Can you work these out from the model? Positions are in its coordinate system, mm. Face numbers are marked on the shaded views. A direction names the side the tool comes from. Give positions to 0.01 mm unless a question says otherwise; leave off trailing zeros. Write each loop counter-clockwise with the first axis right and the second up, starting at its lowest first coordinate (ties: lowest second). Pieces come first, ordered by that corner, then holes.
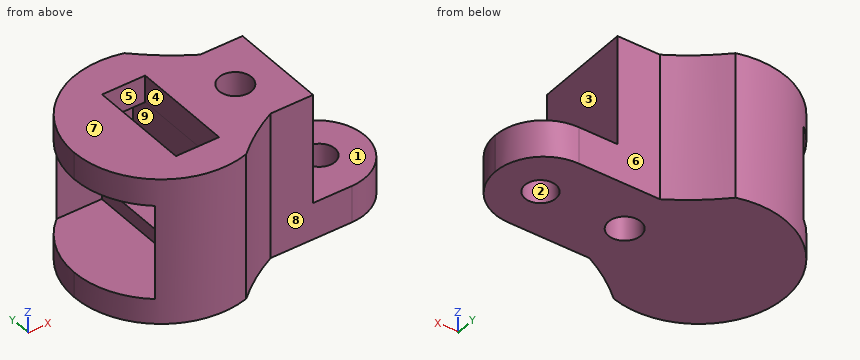
from build123d import *

# Parameters (mm, degrees)
EXTRUDE_1_DEPTH      = 2.2
EXTRUDE_2_DEPTH      = 3.25
SKETCH_3_W           = 50
SKETCH_3_H           = 10.05
EXTRUDE_3_DEPTH      = 3.25
CUT_EXTRUDE_1_DEPTH  = 30
EXTRUDE_4_REACH      = 56.389
SKETCH_6_R           = 5.025
SKETCH_8_R           = 1.675
SKETCH_8_R_2         = 0.84
CUT_EXTRUDE_3_DEPTH  = 55
SKETCH_9_W           = 28.473000816
SKETCH_9_H           = 14.532409192
CUT_EXTRUDE_4_DEPTH  = 3
EXTRUDE_5_DEPTH      = 2.45
SKETCH_11_W          = 12.614203935
SKETCH_11_H          = 10.05
EXTRUDE_6_DEPTH      = 3
SKETCH_12_W          = 36.628466797
SKETCH_12_H          = 15.348537224
CUT_EXTRUDE_5_DEPTH  = 10
SKETCH_13_W          = 5.35
SKETCH_13_H          = 5.35
CUT_EXTRUDE_6_DEPTH  = 14
SKETCH_14_R          = 1.1
CUT_EXTRUDE_7_DEPTH  = 14
SKETCH_15_R          = 1.1
CUT_EXTRUDE_8_DEPTH  = 10
SKETCH_16_R          = 1.625
EXTRUDE_7_DEPTH      = 5.7
SKETCH_17_W          = 19.923143876
SKETCH_17_H          = 15.083058075
CUT_EXTRUDE_9_DEPTH  = 3
SKETCH_18_R          = 1.675
SKETCH_18_R_2        = 1.6
CUT_EXTRUDE_10_DEPTH = 6
CUT_EXTRUDE_11_DEPTH = 10
EXTRUDE_8_DEPTH      = 9.5
EXTRUDE_9_DEPTH      = 15.2
SKETCH_23_W          = 14.793785908
SKETCH_23_H          = 11.59723546
CUT_EXTRUDE_12_DEPTH = 9
SKETCH_25_R          = 1.6
SKETCH_25_R_2        = 1.673969756
CUT_EXTRUDE_13_DEPTH = 20
FILLET_1_R           = 5
SKETCH_26_W          = 0.925753523
SKETCH_26_H          = 16.271734405
EXTRUDE_10_DEPTH     = 15
SKETCH_27_W          = 9.8
SKETCH_27_H          = 13.8
CUT_EXTRUDE_14_DEPTH = 12
SKETCH_28_W          = 4.460954542
SKETCH_28_H          = 10.524407061
CUT_EXTRUDE_15_DEPTH = 12
SKETCH_29_W          = 0.925753523
SKETCH_29_H          = 16.271734405
CUT_EXTRUDE_16_DEPTH = 18
SKETCH_30_W          = 1.5
SKETCH_30_H          = 13.8
EXTRUDE_11_DEPTH     = 3.25


with BuildPart() as part:
    # 草图1 → 凸台-拉伸1 (new body)
    with BuildSketch(Plane.XY):
        with BuildLine():
            Line((1.539836705, 12.851012384), (15.55297303, 14.251012384))
            ThreePointArc((15.55297303, 14.251012384), (17.193415997, 16.063512384), (15.55297303, 17.876012384))
            Line((15.55297303, 17.876012384), (1.500532553, 18.901012384))
            ThreePointArc((1.500532553, 18.901012384), (0.527100583, 19.384612538), (-0.54702697, 19.551012384))
            Line((-0.54702697, 19.551012384), (-0.54702697, 20.901012384))
            Line((-0.54702697, 20.901012384), (19.51277613, 20.901012384))
            Line((19.51277613, 20.901012384), (41.45297303, 20.901012384))
            Line((41.45297303, 20.901012384), (41.45297303, 10.851012384))
            Line((41.45297303, 10.851012384), (-0.54702697, 10.851012384))
            Line((-0.54702697, 10.851012384), (-0.54702697, 12.201012384))
            ThreePointArc((-0.54702697, 12.201012384), (0.54584768, 12.367273294), (1.539836705, 12.851012384))
        make_face()
    extrude(amount=EXTRUDE_1_DEPTH)

    # 草图2 → 凸台-拉伸2 (add)
    with BuildSketch(Plane(origin=(0, 0, 0), x_dir=(-1, 0, 0), z_dir=(0, 0, -1))):
        Polygon((-19.51277613, 10.851012384), (-49.45297303, 10.851012384), (-49.45297303, 20.901012384), (-19.51277613, 20.901012384), (0.54702697, 20.901012384), (0.54702697, 10.851012384), align=None)
    extrude(amount=EXTRUDE_2_DEPTH)

    # 草图3 → 凸台-拉伸3 (add)
    with BuildSketch(Plane.XY.offset(2.2)):
        with Locations((24.45297303, 15.876012384)):
            Rectangle(SKETCH_3_W, SKETCH_3_H)
    extrude(amount=EXTRUDE_3_DEPTH)

    # 草图4 → 切除-拉伸1 (cut, symmetric)
    with BuildSketch(Plane.XY):
        with BuildLine():
            Line((-0.54702697, 19.551012384), (-2.235397712, 16.616091152))
            Line((-2.235397712, 16.616091152), (-1.110896638, 12.310548833))
            Line((-1.110896638, 12.310548833), (-0.54702697, 12.201012384))
            ThreePointArc((-0.54702697, 12.201012384), (0.54584768, 12.367273294), (1.539836705, 12.851012384))
            ThreePointArc((1.539836705, 12.851012384), (2.773180655, 15.88415254), (1.500532553, 18.901012384))
            ThreePointArc((1.500532553, 18.901012384), (0.527100583, 19.384612538), (-0.54702697, 19.551012384))
        make_face()
    extrude(amount=CUT_EXTRUDE_1_DEPTH, both=True, mode=Mode.SUBTRACT)

    # 凸台-拉伸4: up to this face of the body (flat: up to its plane)
    extrude_4_end = Plane(part.part.faces().sort_by_distance((25.407741746, 15.876338503, 5.45))[0])
    # 草图6 → 凸台-拉伸4 (add, up to the picked face)
    with BuildSketch(Plane(origin=(0, 0, -3.25), x_dir=(-1, 0, 0), z_dir=(0, 0, -1)), mode=Mode.PRIVATE) as extrude_4_sk1:
        with Locations(Location((-49.45297303, 15.876012384, 0), (0, 0, 90))):
            Circle(SKETCH_6_R)
    extrude_4_tool1 = split(extrude(extrude_4_sk1.sketch, amount=-EXTRUDE_4_REACH, mode=Mode.PRIVATE), bisect_by=extrude_4_end, keep=Keep.BOTH, mode=Mode.PRIVATE)
    add(extrude_4_tool1.solids().sort_by(Axis((49.452973, 15.876012, -3.25), (0, 0, 1)))[0])

    # 草图8 → 切除-拉伸3 (cut)
    with BuildSketch(Plane(origin=(0, 0, -3.25), x_dir=(-1, 0, 0), z_dir=(0, 0, -1))):
        with Locations((-49.45297303, 15.876012384)):
            Circle(SKETCH_8_R)
        with Locations(Location((-7.95297303, 15.856360308, 0), (0, 0, 180))):
            Circle(SKETCH_8_R_2)
    extrude(amount=-CUT_EXTRUDE_3_DEPTH, mode=Mode.SUBTRACT)

    # 草图9 → 切除-拉伸4 (cut)
    with BuildSketch(Plane(origin=(0, 0, -3.25), x_dir=(-1, 0, 0), z_dir=(0, 0, -1))):
        with Locations((-42.648638606, 15.039406696)):
            Rectangle(SKETCH_9_W, SKETCH_9_H)
    extrude(amount=-CUT_EXTRUDE_4_DEPTH, mode=Mode.SUBTRACT)

    # 草图10 → 凸台-拉伸5 (add)
    with BuildSketch(Plane(origin=(0, 0, 2.2), x_dir=(-1, 0, 0), z_dir=(0, 0, -1))):
        with BuildLine():
            Line((-49.45297303, 20.901012384), (-38.466384114, 20.901012384))
            Line((-38.466384114, 20.901012384), (-38.466384114, 10.851012384))
            Line((-38.466384114, 10.851012384), (-49.45297303, 10.851012384))
            ThreePointArc((-49.45297303, 10.851012384), (-46.217908976, 15.876012384), (-49.45297303, 20.901012384))
        make_face()
    extrude(amount=EXTRUDE_5_DEPTH)

    # 草图11 → 凸台-拉伸6 (add)
    with BuildSketch(Plane(origin=(0, 0, -3.25), x_dir=(-1, 0, 0), z_dir=(0, 0, -1))):
        with Locations((-32.625453647, 15.876012384)):
            Rectangle(SKETCH_11_W, SKETCH_11_H)
    extrude(amount=-EXTRUDE_6_DEPTH)

    # 草图12 → 切除-拉伸5 (cut)
    with BuildSketch(Plane(origin=(0, 0, -3.25), x_dir=(-1, 0, 0), z_dir=(0, 0, -1))):
        with Locations((-5.618322216, 15.103365543)):
            Rectangle(SKETCH_12_W, SKETCH_12_H)
    extrude(amount=-CUT_EXTRUDE_5_DEPTH, mode=Mode.SUBTRACT)

    # 草图13 → 切除-拉伸6 (cut)
    with BuildSketch(Plane.ZY.offset(-23.932555614)):
        with Locations((1.1, 16.124405573)):
            Rectangle(SKETCH_13_W, SKETCH_13_H)
    extrude(amount=-CUT_EXTRUDE_6_DEPTH, mode=Mode.SUBTRACT)

    # 草图14 → 切除-拉伸7 (cut)
    with BuildSketch(Plane(origin=(0, 20.901012384, 0), x_dir=(1, 0, 0), z_dir=(0, 1, 0))):
        with Locations(Location((30.538219594, -1.1, 0), (0, 0, 270))):
            Circle(SKETCH_14_R)
    extrude(amount=-CUT_EXTRUDE_7_DEPTH, mode=Mode.SUBTRACT)

    # 草图15 → 切除-拉伸8 (cut)
    with BuildSketch(Plane.XY.offset(5.45)):
        with Locations((36.879929969, 15.882801083)):
            Circle(SKETCH_15_R)
    extrude(amount=-CUT_EXTRUDE_8_DEPTH, mode=Mode.SUBTRACT)

    # 草图16 → 凸台-拉伸7 (add)
    with BuildSketch(Plane(origin=(0, 0, -0.25), x_dir=(-1, 0, 0), z_dir=(0, 0, -1))):
        with BuildLine():
            Line((-49.45297303, 20.901012384), (23.54702697, 20.901012384))
            ThreePointArc((23.54702697, 20.901012384), (28.57202697, 15.876012384), (23.54702697, 10.851012384))
            Line((23.54702697, 10.851012384), (-49.45297303, 10.851012384))
            Line((-49.45297303, 10.851012384), (-49.45297303, 20.901012384))
        make_face()
        with Locations((23.54702697, 15.876012384)):
            Circle(SKETCH_16_R, mode=Mode.SUBTRACT)
    extrude(amount=-EXTRUDE_7_DEPTH)

    # 草图17 → 切除-拉伸9 (cut)
    with BuildSketch(Plane(origin=(0, 0, -3.25), x_dir=(-1, 0, 0), z_dir=(0, 0, -1))):
        with Locations((-33.178239607, 16.007261263)):
            Rectangle(SKETCH_17_W, SKETCH_17_H)
    extrude(amount=-CUT_EXTRUDE_9_DEPTH, mode=Mode.SUBTRACT)

    # 草图18 → 切除-拉伸10 (cut)
    with BuildSketch(Plane(origin=(0, 0, -0.25), x_dir=(-1, 0, 0), z_dir=(0, 0, -1))):
        with Locations(Location((-49.45297303, 15.876012384, 0), (0, 0, 180))):
            Circle(SKETCH_18_R)
        with Locations((14.84318256, 15.876012384)):
            Circle(SKETCH_18_R_2)
        with BuildLine():
            Line((-31.661597205, 17.303258867), (8.461046927, 17.303258867))
            ThreePointArc((8.461046927, 17.303258867), (9.88829341, 15.876012384), (8.461046927, 14.448765901))
            Line((8.461046927, 14.448765901), (-31.661597205, 14.448765901))
            ThreePointArc((-31.661597205, 14.448765901), (-33.088843687, 15.876012384), (-31.661597205, 17.303258867))
        make_face()
    extrude(amount=-CUT_EXTRUDE_10_DEPTH, mode=Mode.SUBTRACT)

    # 草图19 → 切除-拉伸11 (cut)
    with BuildSketch(Plane(origin=(0, 0, -0.25), x_dir=(-1, 0, 0), z_dir=(0, 0, -1))):
        Polygon((12.697516125, 20.901012384), (-60.999534113, 39.375054119), (-58.738783937, -10.22846445), (12.697516125, 10.851012384), (10.156545193, 10.851012384), (10.156545193, 20.901012384), align=None)
    extrude(amount=-CUT_EXTRUDE_11_DEPTH, mode=Mode.SUBTRACT)

    # 草图21 → 凸台-拉伸8 (add)
    with BuildSketch(Plane.XY.offset(5.45)):
        with BuildLine():
            Line((-23.54702697, 20.901012384), (-12.697516125, 20.901012384))
            ThreePointArc((-12.697516125, 20.901012384), (-9.87974938, 15.876012384), (-12.697516125, 10.851012384))
            Line((-12.697516125, 10.851012384), (-23.54702697, 10.851012384))
            ThreePointArc((-23.54702697, 10.851012384), (-28.57202697, 15.876012384), (-23.54702697, 20.901012384))
        make_face()
    extrude(amount=EXTRUDE_8_DEPTH)

    # 草图22 → 凸台-拉伸9 (add)
    with BuildSketch(Plane(origin=(0, 0, -0.25), x_dir=(-1, 0, 0), z_dir=(0, 0, -1))):
        with BuildLine():
            Line((23.54702697, 20.901012384), (26.601137036, 16.368267617))
            Line((26.601137036, 16.368267617), (23.54702697, 10.851012384))
            ThreePointArc((23.54702697, 10.851012384), (26.137365286, 9.34674893), (28.497704507, 7.502444211))
            ThreePointArc((28.497704507, 7.502444211), (40.025732832, 16.109516943), (28.556434004, 24.794695265))
            ThreePointArc((28.556434004, 24.794695265), (26.173914365, 22.690658492), (23.54702697, 20.901012384))
        make_face()
    extrude(amount=-EXTRUDE_9_DEPTH)

    # 草图23 → 切除-拉伸12 (cut, symmetric)
    with BuildSketch(Plane(origin=(-10.156545193, 0, 0), x_dir=(0, 0, -1), z_dir=(1, 0, 0))):
        with Locations((-10.971714959, 15.6975909)):
            Rectangle(SKETCH_23_W, SKETCH_23_H)
    extrude(amount=CUT_EXTRUDE_12_DEPTH, both=True, mode=Mode.SUBTRACT)

    # 草图25 → 切除-拉伸13 (cut)
    with BuildSketch(Plane(origin=(0, 0, -0.25), x_dir=(-1, 0, 0), z_dir=(0, 0, -1))):
        with Locations((14.84318256, 15.876012384)):
            Circle(SKETCH_25_R)
        with Locations((23.54702697, 15.876012384)):
            Circle(SKETCH_25_R_2)
    extrude(amount=-CUT_EXTRUDE_13_DEPTH, mode=Mode.SUBTRACT)

    # 圆角1
    fillet_1_edges = [part.edges().sort_by_distance(p)[0] for p in [
        (-10.156545193, 10.851012384, 1.662411002),
        (-10.156545193, 20.901012384, 1.662411002),
    ]]
    fillet(fillet_1_edges, radius=FILLET_1_R)

    # 草图26 → 凸台-拉伸10 (add)
    with BuildSketch(Plane(origin=(0, 0, -0.25), x_dir=(-1, 0, 0), z_dir=(0, 0, -1))):
        with Locations((40.488609594, 16.108824789)):
            Rectangle(SKETCH_26_W, SKETCH_26_H)
    extrude(amount=-EXTRUDE_10_DEPTH)

    # 草图27 → 切除-拉伸14 (cut)
    with BuildSketch(Plane.ZY.offset(40.951486355)):
        with Locations((7.257156835, 16.078298666)):
            Rectangle(SKETCH_27_W, SKETCH_27_H)
    extrude(amount=-CUT_EXTRUDE_14_DEPTH, mode=Mode.SUBTRACT)

    # 草图28 → 切除-拉伸15 (cut)
    with BuildSketch(Plane(origin=(0, 0, 12.157156835), x_dir=(-1, 0, 0), z_dir=(0, 0, -1))):
        with Locations((31.184244341, 16.001788247)):
            Rectangle(SKETCH_28_W, SKETCH_28_H)
    extrude(amount=-CUT_EXTRUDE_15_DEPTH, mode=Mode.SUBTRACT)

    # 草图29 → 切除-拉伸16 (cut)
    with BuildSketch(Plane(origin=(0, 0, -0.25), x_dir=(-1, 0, 0), z_dir=(0, 0, -1))):
        with Locations((40.488609594, 16.108824789)):
            Rectangle(SKETCH_29_W, SKETCH_29_H)
    extrude(amount=-CUT_EXTRUDE_16_DEPTH, mode=Mode.SUBTRACT)

    # 草图30 → 凸台-拉伸11 (add)
    with BuildSketch(Plane.ZY.offset(28.951486355)):
        with Locations((3.107156835, 16.078298666)):
            Rectangle(SKETCH_30_W, SKETCH_30_H)
    extrude(amount=EXTRUDE_11_DEPTH)


solid = part.part
(1) For the marked faces 5, 6, 7, 8 and 9, which set-ups out of +Z, -Z, +X, -X, +Y, -Y let a thin tool reach every point of the face, with its end or its side?
Returned:
face 5: +Z
face 6: +Z, -Z, +X, +Y
face 7: +Z, +X, -X, +Y, -Y
face 8: +Z, -Z, +X, -Y
face 9: -X
(2) Imagine slicing it at A-A, the plane y = 15.25. Give the number of separate pieces and of enclosed holes in the cut face, plus the area to 3 significant figures.
Returned:
separate pieces: 4
enclosed holes: 0
area: 177 mm2
(3) If we mould it in two halves opening along X, with no side actions, what happens to the marked faces 1, 2, 3 and 4? For each: +X half, -X half, draft (parallel to the pull), parting line (faces both ways), or undercut.
Returned:
face 1: draft
face 2: undercut
face 3: +X half
face 4: undercut
(4) If I drill on L1, parallel to Z at x = -37.25, y = 20.75; L2, parallel to Z at x = -29.5, y = 22.5; L3, parallel to Y at x = -31.25, z = 11, over which ranges is the centre line in solid material (lowest first)?
Returned:
L1: z = -0.25 to 2.36, 12.16 to 14.95
L2: z = -0.25 to 3.86, 12.16 to 14.95
L3: y = 7.14 to 9.18, 22.98 to 25.14
(5) Imagine slicing it at C-C, the plane z = 7.5. Write out the boundary of the cut face in (x, y), plus the area to 3 significant figures.
Returned:
outline: (-36.88, 22.98) - (-28.95, 22.98) - (-28.95, 9.18) - (-36.73, 9.18) arc R9 ccw to (-28.5, 7.5) arc R21.86 cw to (-23.55, 10.85) - (-19.16, 10.85) - (-19.16, 20.9) - (-23.55, 20.9) arc R25.37 cw to (-28.56, 24.79) arc R9 ccw to start; hole circle Ø3.35 at (-23.55, 15.88)
area: 134 mm2
(6) Will these pins go through, and if not, where does the flat tip stop? P1, Ø0.8, axis at y = 15.5, z = 13.5, coming from the +X side; P2, Ø1.4, axis at y = 18.5, z = 13.5, coming from the -X side; P3, Ø2.5, axis at x = -18.5, z = 8, coming from the -Y side.
Returned:
P1: stops at x = -19.16
P2: stops at x = -39.87
P3: stops at y = 10.85
(7) Imagine slicing it at B-B, the plane x = -35.5. Write out the boundary of the cut face in (y, z), plus the area to 3 significant figures.
Returned:
outline: (8.33, -0.25) - (23.95, -0.25) - (23.95, 14.95) - (8.33, 14.95) - close; hole (9.18, 2.36) - (22.98, 2.36) - (22.98, 12.16) - (9.18, 12.16) - close
area: 102 mm2
